from build123d import *

# Parameters (mm, degrees)
SKETCH1_R           = 1.27
BOSS_EXTRUDE2_DEPTH = 1.5875
SKETCH3_R           = 4.191
CUT_EXTRUDE1_DEPTH  = 2.54
SKETCH4_R           = 1
SKETCH4_R_2         = 0.999998
CUT_EXTRUDE2_DEPTH  = 2.54


with BuildPart() as part:
    # Sketch1 → Boss-Extrude2 (new body)
    with BuildSketch(Plane(origin=(0, 0, 0), x_dir=(1, 0, 0), z_dir=(0, 1, 0))):
        Polygon((-41.794385987, 35.56), (0, 11.43), (0, 0), (17.78, 0), (17.78, -67.587878735), (33.02, -67.587878735), (33.02, 0), (50.8, 0), (50.8, 11.43), (92.594385987, 35.56), (84.974385987, 48.758227154), (43.18, 24.628227154), (7.62, 24.628227154), (-34.174385987, 48.758227154), align=None)
        with Locations(Location((36.398522628, 11.914121265, 0), (0, 0, 270))):
            Circle(SKETCH1_R, mode=Mode.SUBTRACT)
        with Locations(Location((14.401477372, 11.914121265, 0), (0, 0, 270))):
            Circle(SKETCH1_R, mode=Mode.SUBTRACT)
        with Locations(Location((25.4, -7.135878735, 0), (0, 0, 270))):
            Circle(SKETCH1_R, mode=Mode.SUBTRACT)
    extrude(amount=BOSS_EXTRUDE2_DEPTH)

    # Sketch3 → Cut-Extrude1 (cut)
    with BuildSketch(Plane(origin=(0, 1.5875, 0), x_dir=(1, 0, 0), z_dir=(0, 1, 0))):
        with Locations(Location((28.778522628, 17.627987154, 0), (0, 0, 270))):
            Circle(SKETCH3_R)
    extrude(amount=-CUT_EXTRUDE1_DEPTH, mode=Mode.SUBTRACT)

    # Sketch4 → Cut-Extrude2 (cut)
    with BuildSketch(Plane(origin=(0, 1.5875, 0), x_dir=(1, 0, 0), z_dir=(0, 1, 0))):
        with Locations(Location((25.4, -59.967878735, 0), (0, 0, 270))):
            Circle(SKETCH4_R)
        with Locations(Location((25.4, -47.267878735, 0), (0, 0, 270))):
            Circle(SKETCH4_R_2)
        with Locations(Location((-20.386749782, 31.999113577, 0), (0, 0, 270))):
            Circle(SKETCH4_R)
        with Locations(Location((-31.38527241, 38.349113577, 0), (0, 0, 270))):
            Circle(SKETCH4_R)
        with Locations(Location((82.18527241, 38.349113577, 0), (0, 0, 270))):
            Circle(SKETCH4_R)
        with Locations(Location((71.186749782, 31.999113577, 0), (0, 0, 270))):
            Circle(SKETCH4_R)
    extrude(amount=-CUT_EXTRUDE2_DEPTH, mode=Mode.SUBTRACT)


solid = part.part
Part model, mm, in its own coordinate system. A direction names the side the tool comes from. Coordinates: 2 decimals unless noted, no trailing zeros. Order: outer loops, then holes, each group sorted by start corner. A loop starts at its lowest first (then second) coordinate and runs counter-clockwise, first axis right, second up. Notation, with made-up numbers: M 28,23 L 69,23 A25 ccw 69,52 Z; hole C -19.75,75.25 d11. An arc over 180 degrees is marked long. One line per question, with ' | ' between items.
Q1. Drill centre lines: line 1 (X direction, y = 0.45, z = -31.5); line 2 (Z direction, x = 23, y = 1); line 3 (X direction, y = 0.5, z = 26). Where is each one in solid material? Low to high.
A:
line 1: x = -34.76 to -21.25, -19.52 to -4.28, 55.08 to 70.32, 72.05 to 85.56 | line 2: z = -24.63 to 67.59 | line 3: x = 17.78 to 33.02
Q2. Slice it at A-A (z = -19). Give the cut face in (x, y), and give its area (3 significant figures).
A:
outline: M -13.11,0 L 24.82,0 L 24.82,1.59 L -13.11,1.59 Z; M 32.74,0 L 63.91,0 L 63.91,1.59 L 32.74,1.59 Z | area: 110 mm^2
Q3. 3-axis set-ups, long thin cutter, end or side, ignore diameter. For faces 1 (the face through (88.838, 0.783, -42.067)), 2 (the face through (64.37, 0.78, -36.86)): which of +Z, -Z, +X, -X, +Y, -Y reach the whole face in a straight line?
A:
face 1: -Z, +X, +Y, -Y | face 2: -Z, +Y, -Y
Q4. Slice it at D-D (x = 67). Give the cut face in (y, z), and give its area (3 significant figures).
A:
outline: M 0,-38.38 L 1.59,-38.38 L 1.59,-20.78 L 0,-20.78 Z | area: 27.9 mm^2
Q5. Two-plate mould, pull along Z, no slides. Class faces 3 (the face through (-37.93, 0.78, -42.25)), 4 (the face through (-21.19, 0.783, -23.664)), 5 (the face through (27.17, 0.8, -13.76)), 6 (the face through (25, 0, -8)): +Z half, -Z half, draft (parallel to the pull), parting line (faces both ways), or undercut.
A:
face 3: -Z half | face 4: +Z half | face 5: undercut | face 6: draft
Q6. Slice it at C-C (z = -6). Give the cut face in (x, y).
A:
outline: M 0,0 L 50.8,0 L 50.8,1.59 L 0,1.59 Z
Q7. Pin check, flat tips, straight feed: P1, Ø0.5, axis at y = 0.5, z = -6, coming from the -X side; P2, Ø0.8, axis at x = 9.5, y = 0.5, coming from the +Z side. Stop position of each tip, or through.
A:
P1: stops at x = 0 | P2: stops at z = 0
Q8. Slice it at B-B (y = 0.9). Count the separate pieces of the cut face and the enclosed holes in it, and give its area (3 significant figures).
A:
separate pieces: 1 | enclosed holes: 10 | area: 3,560 mm^2
